```python
from build123d import *

# Parameters (mm, degrees)
ESQUISSE1_W             = 49
ESQUISSE1_H             = 40
BOSS_EXTRU_1_DEPTH      = 4
ESQUISSE2_W             = 4
ESQUISSE2_H             = 40
BOSS_EXTRU_2_DEPTH      = 14
ESQUISSE3_R             = 3
ENL_V_MAT_EXTRU_1_DEPTH = 4
ESQUISSE4_R             = 3
ESQUISSE4_R_2           = 2
ENL_V_MAT_EXTRU_2_DEPTH = 5


with BuildPart() as part:
    # Esquisse1 → Boss.-Extru.1 (new body)
    with BuildSketch(Plane.XY):
        with Locations((-2.585864486, -2.70959596)):
            Rectangle(ESQUISSE1_W, ESQUISSE1_H)
    extrude(amount=BOSS_EXTRU_1_DEPTH)

    # Esquisse2 → Boss.-Extru.2 (add)
    with BuildSketch(Plane.XY.offset(4)):
        with Locations((19.914135514, -2.70959596)):
            Rectangle(ESQUISSE2_W, ESQUISSE2_H)
    extrude(amount=BOSS_EXTRU_2_DEPTH)

    # Esquisse3 → Enlèv. mat.-Extru.1 (cut)
    with BuildSketch(Plane(origin=(21.914135514, 0, 0), x_dir=(0, 0, -1), z_dir=(1, 0, 0))):
        with Locations(Location((-11, 8.04040404, 0), (0, 0, 90))):  # turned: the seam where the file's is
            Circle(ESQUISSE3_R)
        with Locations(Location((-11, -12.45959596, 0), (0, 0, 90))):  # turned: the seam where the file's is
            Circle(ESQUISSE3_R)
    extrude(amount=-ENL_V_MAT_EXTRU_1_DEPTH, mode=Mode.SUBTRACT)

    # Esquisse4 → Enlèv. mat.-Extru.2 (cut, through all)
    with BuildSketch(Plane.XY.offset(4)):
        with Locations((-7.085864486, -2.70959596)):
            Circle(ESQUISSE4_R)
        with Locations((-22.585864486, 12.79040404)):
            Circle(ESQUISSE4_R_2)
        with Locations((8.414135514, 12.79040404)):
            Circle(ESQUISSE4_R_2)
        with Locations((8.414135514, -18.20959596)):
            Circle(ESQUISSE4_R_2)
        with Locations((-22.585864486, -18.20959596)):
            Circle(ESQUISSE4_R_2)
    extrude(amount=-ENL_V_MAT_EXTRU_2_DEPTH, mode=Mode.SUBTRACT)


solid = part.part
```
Can you work these out from the model? Positions are in its coordinate system, mm. A direction names the side the tool comes from. Give positions to 0.01 mm unless a question says otherwise; leave off trailing zeros. Loops run counter-clockwise (first coordinate to the right, second up) from the corner with the lowest first, then second, coordinate; pieces in that order, holes last. Notation, with made-up numbers: M -30.5,21.5 L -22.5,21.5 A27 cw -22.5,60.5 Z; hole C 44,-32 d10. An arc over 180 degrees is marked long. Use CSV: the item, a comma, the result in double quotes. Start each with the question number.
1. Imagine slicing it at B-B, the plane x = -6. Write out the boundary of the cut face in (y, z), plus the area to 3 significant figures.
2. Imagine slicing it at C-C, the plane y = -0.5. Write out the boundary of the cut face in (x, z).
3. On a 3-axis mill with a long thin cutter (end or side, diameter ignored), from which of +Z, -Z, +X, -X, +Y, -Y can I reach the whole of each face in a straight line? I mean faces 1 (the face through (17.914, -3, 11)), 2 (the face through (19.942, -15.457, 11.132)). Say none if no direction works.
4. Imagine slicing it at D-D, the plane x = -22.5. Write out the boundary of the cut face in (y, z), plus the area to 3 significant figures.
5. Imagine slicing it at A-A, the plane z = 11. Write out the boundary of the cut face in (x, y), plus the area to 3 significant figures.
6. If we mould it in two halves opening along X, with no side actions, what happens to faces 3 (the face through (1, -22.71, 3)), 4 (the face through (-24.17, -19.43, 2.03)), 5 (the face through (-27.086, -3, 2))? For each: released by +X, released by -X, zero draft, split by the parting line, or undercut.
7. If I drill on L1, parallel to X at y = -19.5, z = 6.5; L2, parallel to Y at x = 7, z = 3; L3, parallel to X at y = -1.5, z = 3.25, over which ranges is the centre line in solid material (lowest first)?
8. For P1, Ø4.5, axis at x = -22.59, y = -18.21, coming from the +Z side; P2, Ø7, axis at y = 4.5, z = 14.5, coming from the -X side, each with a flat end and sliding along its axis, tell me the tip position at first contact or that it passes through.
Response values:
1,outline,"M -22.71,0 L -5.51,0 L -5.51,4 L -22.71,4 Z; M 0.09,0 L 17.29,0 L 17.29,4 L 0.09,4 Z"
1,area,"138 mm^2"
2,outline,"M -27.09,0 L -9.12,0 L -9.12,4 L -27.09,4 Z; M -5.06,0 L 21.91,0 L 21.91,18 L 17.91,18 L 17.91,4 L -5.06,4 Z"
3,face 1,"+Z, -X, +Y, -Y"
3,face 2,"+X, -X"
4,outline,"M -22.71,0 L -20.21,0 L -20.21,4 L -22.71,4 Z; M -16.21,0 L 10.79,0 L 10.79,4 L -16.21,4 Z; M 14.79,0 L 17.29,0 L 17.29,4 L 14.79,4 Z"
4,area,"128 mm^2"
5,outline,"M 17.91,-22.71 L 21.91,-22.71 L 21.91,-15.46 L 17.91,-15.46 Z; M 17.91,-9.46 L 21.91,-9.46 L 21.91,5.04 L 17.91,5.04 Z; M 17.91,11.04 L 21.91,11.04 L 21.91,17.29 L 17.91,17.29 Z"
5,area,"112 mm^2"
6,face 3,"zero draft"
6,face 4,"undercut"
6,face 5,"released by -X"
7,L1,"17.91 to 21.91"
7,L2,"-22.71 to -19.62, -16.8 to 11.38, 14.2 to 17.29"
7,L3,"-27.09 to -9.83, -4.34 to 21.91"
8,P1,"z = 4"
8,P2,"x = 17.91"
